Geometry check sheet. Reference: drawing and pictorial views, mm from the part's lowest x, y, z. A direction names the side the tool comes from. Give positions to 0.01 mm unless a question says otherwise; leave off trailing zeros. Order: outer loops, then holes, each group sorted by start corner. A loop starts at its lowest first (then second) coordinate and runs counter-clockwise, first axis right, second up. Notation, with made-up numbers: (-29.75, 76.5) -> (8.25, 76.5) arc R16 ccw to (8.25, 94.5) -> close; hole circle Ø6 at (81, -36.5). An arc over 180 degrees is marked (long way). Write each question's results on one line, items separated by ' | '. Start each with the question number.
1. Set-up check for the marked faces 5 and 6: record each of +Z, -Z, +X, -X, +Y, -Y from which the full face is reachable in a straight line by a thin tool's end or side.
2. Mould release check, pull along X, two halves, no side actions. Record for the marked faces 1, 2, 3 and 4: +X half, -X half, draft (parallel to the pull), parting line (faces both ways), or undercut.
3. Cross-section at A-A, the plane z = 1.1. Enter the section's corners in (x, y).
4. Material ranges on L1, parallel to Y at x = 3, z = 1.25; L2, parallel to Y at x = 5.1, z = 1.3; L3, parallel to Y at x = 1.8, z = 0.7 (1 decimal), recorded low to high. Write a range as from..to.
5. Cross-section at D-D, the plane x = 5.1. Enter the section's corners in (y, z), then the cut area to 3 significant figures.
6. Depth check by flat-ended pin: pin 1 Ø1 at (y, z) = (18, 0.5) entering from -X. Enter the tip coordinate at first touch or a pass-through.
7. Cross-section at C-C, the plane x = 3. Enter the section's corners in (y, z).
8. Cross-section at B-B, the plane y = 34. Enter the section's corners in (x, z).
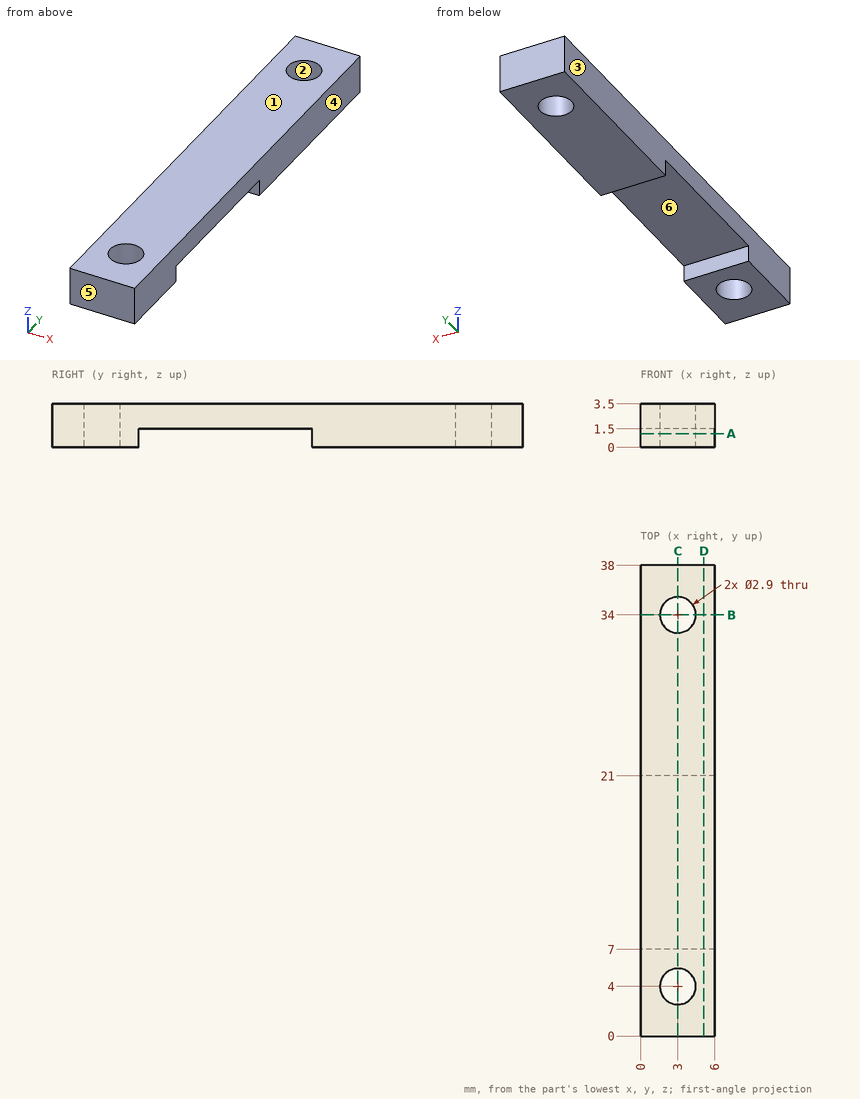
Results below:
1) face 5: +Z, -Z, +X, -X, -Y | face 6: -Z, +X, -X
2) face 1: draft | face 2: undercut | face 3: -X half | face 4: +X half
3) outline: (0, 0) -> (6, 0) -> (6, 7) -> (0, 7) -> close; (0, 21) -> (6, 21) -> (6, 38) -> (0, 38) -> close; hole circle Ø2.9 at (3, 4); hole circle Ø2.9 at (3, 34)
4) L1: y = 0..2.55, 5.45..7, 21..32.55, 35.45..38 | L2: y = 0..7, 21..38 | L3: y = 0..3.2, 4.8..7, 21..33.2, 34.8..38
5) outline: (0, 0) -> (7, 0) -> (7, 1.5) -> (21, 1.5) -> (21, 0) -> (38, 0) -> (38, 3.5) -> (0, 3.5) -> close | area: 112 mm²
6) pin 1: passes through
7) outline: (0, 0) -> (2.55, 0) -> (2.55, 3.5) -> (0, 3.5) -> close; (5.45, 0) -> (7, 0) -> (7, 1.5) -> (21, 1.5) -> (21, 0) -> (32.55, 0) -> (32.55, 3.5) -> (5.45, 3.5) -> close; (35.45, 0) -> (38, 0) -> (38, 3.5) -> (35.45, 3.5) -> close
8) outline: (0, 0) -> (1.55, 0) -> (1.55, 3.5) -> (0, 3.5) -> close; (4.45, 0) -> (6, 0) -> (6, 3.5) -> (4.45, 3.5) -> close
